Part model, mm, in its own coordinate system. Face numbers are marked on the shaded views. A direction names the side the tool comes from. Give positions to 0.01 mm unless a question says otherwise; leave off trailing zeros. Order: outer loops, then holes, each group sorted by start corner. A loop starts at its lowest first (then second) coordinate and runs counter-clockwise, first axis right, second up. Notation, with made-up numbers: (77.25, 8) - (87.25, 8) arc R12 cw to (87.25, 31) - close; hole circle Ø7 at (78.5, 61). An arc over 180 degrees is marked (long way). Use a Markdown table: item, result. Add a question column.
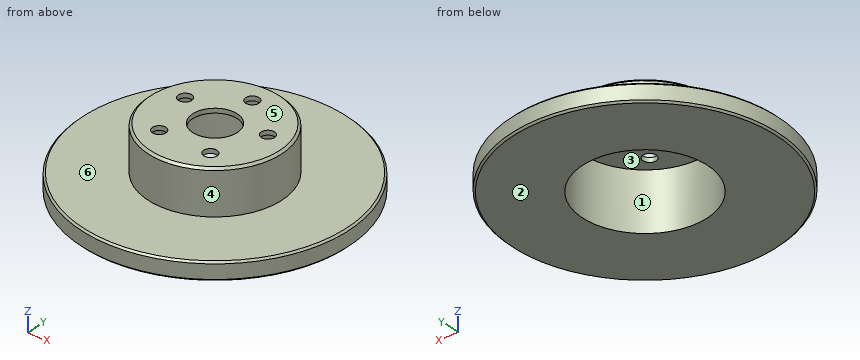
Autodesk Fusion 360 part; units mm, degrees
sketch "Sketch1" plane through (0, 0, 0) normal (0, 0, 1) x (1, 0, 0) in component "Disk"
  circle A0 centre (0, 0) radius 150
  dimension "d1" = 300
extrude "Extrude1" add sketch "Sketch1" along normal blind 20 in component "Disk"
sketch "Sketch2" plane through (0, 0, 20) normal (0, 0, 1) x (1, 0, 0) in component "Disk"
  circle A0 centre (0, 0) radius 150
  circle A1 centre (0, 0) radius 75
  dimension "d4" = 150
extrude "Extrude2" add sketch "Sketch2" along normal blind 50 contours A1 in component "Disk"
sketch "Sketch3" plane through (0, 0, 0) normal (0, 0, -1) x (-1, 0, 0) in component "Disk"
  circle A0 centre (0, 0) radius 150
  circle A1 centre (0, 0) radius 75
  circle A2 centre (0, 0) radius 70
  dimension "d7" = -5
extrude "Extrude3" cut sketch "Sketch3" against normal up to surface (65 mm away) contours A2 in component "Disk"
chamfer "Chamfer1" distance 2.5 angle 45 1 edges at (-69.9246, -27.1212, 70) in component "Disk"
chamfer "Chamfer2" distance 2 angle 45 2 edges at (-139.8491, -54.2423, 20) (-139.8491, -54.2423, 0) in component "Disk"
sketch "Sketch4" plane through (0, 0, 70) normal (0, 0, 1) x (1, 0, 0) in component "Disk"
  circle A0 centre (0, 0) radius 72.5
  circle A1 centre (0, 0) radius 25
  dimension "d12" = 50
extrude "Extrude4" cut sketch "Sketch4" against normal up to surface (5 mm away) contours A1 in component "Disk"
sketch "Sketch5" plane through (0, 0, 70) normal (0, 0, 1) x (1, 0, 0) in component "Disk"
  circle A0 centre (0, 0) radius 25
  circle A1 centre (0, 0) radius 72.5
  point P0 (0, 50)
  dimension "d15" = 50
hole "Hole1" at (0, 50, 70) direction (0, 0, -1) diameter 15 depth 5 tip angle 118 in component "Disk"
pattern_circular "C-Pattern1" count 5 over 360 about axis through (0, 0, 70) along (0, 0, -1) of "Hole1" in component "Disk"
component "Disk" placed x (1, 0, 0) y (0, 1, 0) z (0, 0, 1) at (0, 0, 0)
1. Drill centre lines: probe 1 along Y at (x, z) = (0, 66.2); probe 2 along Y at (x, z) = (0, 67.75); probe 3 along X at (y, z) = (13, 40.5). Where is each one in solid material? Low to high. Write a range as [from, to].
2. Cut at C-C (z = 10.5). Write the cut outline in (x, y).
3. Cut at A-A (y = 0). Write the cut outline in (x, z).
4. Cut at B-B (x = 0). Write the cut outline in (y, z), plus the area to 3 significant figures.
5. Pin check, flat tips, straight feed: P1, Ø1, axis at x = 74, y = 3, coming from the -Z side; P2, Ø1.5, axis at x = 63.5, z = 35, coming from the -Y side; P3, Ø6, axis at x = 36.5, y = -84, coming from the +Z side; P4, Ø6, axis at x = 57.5, z = 32.5, coming from the +Y side. Stop position of each tip, or through.
6. Cut at D-D (z = 31). Write the cut outline in (x, y).
7. Mould opens along Y. For the marked faces 1, 2, 3 and 4 say: released by +Y, released by -Y, zero draft, split by the parting line, or undercut.
8. Tool access for the marked faces 5 and 6: list every direction of +Z, -Z, +X, -X, +Y, -Y with a clear straight run to the whole face (end or side of a thin tool).
Responses:
| question | item | result |
|---|---|---|
| 1 | probe 1 | y = [-75, -25], [25, 42.5], [57.5, 75] |
| 1 | probe 2 | y = [-74.75, -25], [25, 42.5], [57.5, 74.75] |
| 1 | probe 3 | x = [-73.86, -68.78], [68.78, 73.86] |
| 2 | outline | circle Ø300 at (0, 0); hole circle Ø140 at (0, 0) |
| 3 | outline | (-150, 2) - (-148, 0) - (-70, 0) - (-70, 65) - (-25, 65) - (-25, 70) - (-72.5, 70) - (-75, 67.5) - (-75, 20) - (-148, 20) - (-150, 18) - close; (25, 65) - (70, 65) - (70, 0) - (148, 0) - (150, 2) - (150, 18) - (148, 20) - (75, 20) - (75, 67.5) - (72.5, 70) - (25, 70) - close |
| 4 | outline | (-150, 2) - (-148, 0) - (-70, 0) - (-70, 65) - (-25, 65) - (-25, 70) - (-72.5, 70) - (-75, 67.5) - (-75, 20) - (-148, 20) - (-150, 18) - close; (25, 65) - (42.5, 65) - (42.5, 70) - (25, 70) - close; (57.5, 65) - (70, 65) - (70, 0) - (148, 0) - (150, 2) - (150, 18) - (148, 20) - (75, 20) - (75, 67.5) - (72.5, 70) - (57.5, 70) - close |
| 4 | area | 4,060 mm² |
| 5 | P1 | stops at z = 0 |
| 5 | P2 | stops at y = -41.08 |
| 5 | P3 | stops at z = 20 |
| 5 | P4 | stops at y = 51.52 |
| 6 | outline | circle Ø150 at (0, 0); hole circle Ø140 at (0, 0) |
| 7 | face 1 | undercut |
| 7 | face 2 | zero draft |
| 7 | face 3 | undercut |
| 7 | face 4 | split by the parting line |
| 8 | face 5 | +Z, +X, -X, +Y, -Y |
| 8 | face 6 | +Z |
